Could you check a few things on this model? Use its own coordinates, in mm. Face numbers are marked on the shaded views. Coordinates: 2 decimals unless noted, no trailing zeros. Loops run counter-clockwise (first coordinate to the right, second up) from the corner with the lowest first, then second, coordinate; pieces in that order, holes last.
1) Imagine slicing it at A-A on y = 0. Please give me the cut outline in (x, z).
2) If I drill on line 1 along X through (y, z) = (1, -2.75); line 2 along Y through (x, z) = (0, 1.5); line 3 along X through (y, z) = (4.5, 2.5), over which ranges is the centre line in solid material (lowest first)?
3) Thinking about a two-plate mould opening in X: for the marked faces 1 and 2, which applies, released by +X, released by -X, zero draft, split by the parting line, or undercut?
4) Will these pins go through, and if not, where does the flat tip stop? P1, Ø1.5, axis at x = 10, z = 3, coming from the -Y side; P2, Ø4, axis at x = -3, y = -3, coming from the +Z side; P3, Ø8, axis at x = 2, y = 10, coming from the -Z side.
5) Imagine slicing it at D-D on z = 3. Please give me the cut outline in (x, y).
6) Imagine slicing it at C-C on z = 0.5. Please give me the cut outline in (x, y), plus the area to 3 significant figures.
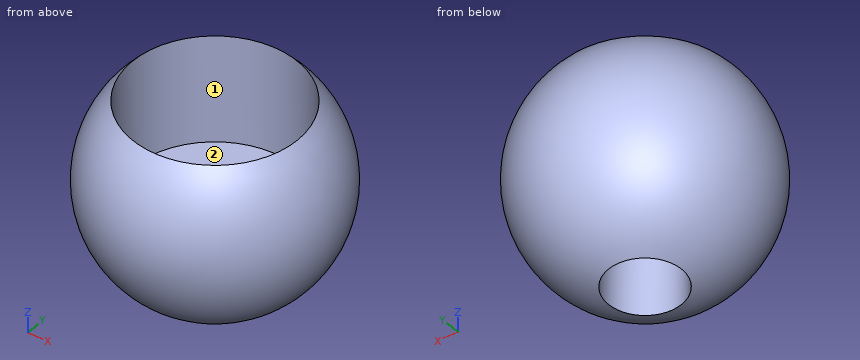
```python
from build123d import *

# Parameters (mm, degrees)
CYLINDER001_R     = 9
CYLINDER001_DEPTH = 15
CYLINDER_R        = 4
CYLINDER_DEPTH    = 30


with BuildPart() as cylinder001:
    # Cylinder001 → Cylinder001 (new body)
    with BuildSketch(Plane.XY.offset(-3)):
        Circle(CYLINDER001_R)
    extrude(amount=CYLINDER001_DEPTH)


with BuildPart() as fusion:
    # Cylinder → Cylinder (new body)
    with BuildSketch(Plane.XY.offset(-15)):
        Circle(CYLINDER_R)
    extrude(amount=CYLINDER_DEPTH)

    # Fusion: union Cylinder001
    add(cylinder001.part)


with BuildPart() as final:
    # Sphere → Sphere (revolve)
    with BuildSketch(Plane.XZ):
        with BuildLine():
            ThreePointArc((0, -12.5), (12.5, 0), (0, 12.5))
            Line((0, 12.5), (0, -12.5))
        make_face()
    revolve(axis=Axis((0, 0, 0), (0, 0, 1)))

    # Cut: cut Fusion
    add(fusion.part, mode=Mode.SUBTRACT)


solid = final.part
```
Filled in:
1. outline: (-9, -3) - (-9, 8.67) arc R12.5 ccw to (-4, -11.84) - (-4, -3) - close; (4, -11.84) arc R12.5 ccw to (9, 8.67) - (9, -3) - (4, -3) - close
2. line 1: x = -12.15 to -8.94, 8.94 to 12.15
2. line 2: y = -12.41 to -9, 9 to 12.41
2. line 3: x = -11.39 to -7.79, 7.79 to 11.39
3. face 1: undercut
3. face 2: undercut
4. P1: stops at y = -7.9
4. P2: stops at z = -3
4. P3: stops at z = -10.86
5. outline: circle Ø24.27 at (0, 0); hole circle Ø18 at (0, 0)
6. outline: circle Ø24.98 at (0, 0); hole circle Ø18 at (0, 0)
6. area: 236 mm2
